For this review, use the dimensioned drawing (mm, ordinates from the lowest corner) and the shaded views. A direction names the side the tool comes from. Coordinates: 2 decimals unless noted, no trailing zeros. Loops run counter-clockwise (first coordinate to the right, second up) from the corner with the lowest first, then second, coordinate; pieces in that order, holes last. Notation, with made-up numbers: (7.25, 64.5) - (24.25, 64.5) arc R16 cw to (24.25, 91.5) - close; hole circle Ø8 at (54.5, -5.75). An arc over 180 degrees is marked (long way). Answer in a Markdown table with one row per item. Add a question column.
(1) Machinability: for the marked faces 5, 6, 7 and 8, which of the approach directions +Z, -Z, +X, -X, +Y, -Y give a long, thin tool a straight path to every point of the face, cutting with its end or side? Answer none if there is none.
(2) For line 1 along Y through (x, z) = (2, 7.75); line 2 along X through (y, z) = (47.5, 9), list the stretches that pass through material, from the lowest coordinate up.
(3) We need section B-B on z = 3. Write out the cut boundary in (x, y), plus the area to 3 significant figures.
(4) Mouldability with a two-part tool opening along Y and no side actions: class the marked faces 1, 2, 3 and 4 as +Y half, -Y half, draft (parallel to the pull), parting line (faces both ways), or undercut.
(5) We need section A-A on x = 3. Write out the cut boundary in (y, z), plus the area to 3 significant figures.
(6) We need section C-C on z = 7.25. Write out the cut boundary in (x, y).
(7) We need section D-D on y = 43. Write out the cut boundary in (x, z), plus the area to 3 significant figures.
(8) For P1, Ø1.5, axis at x = 16.5, z = 11, coming from the +Y side; P2, Ø5.5, axis at y = 48.5, z = 11.5, coming from the +X side; P3, Ø5.5, axis at x = 1.5, y = 40, coming from the -Z side, all flat-tipped, find the tip position at first contact; note any pin that passes through.
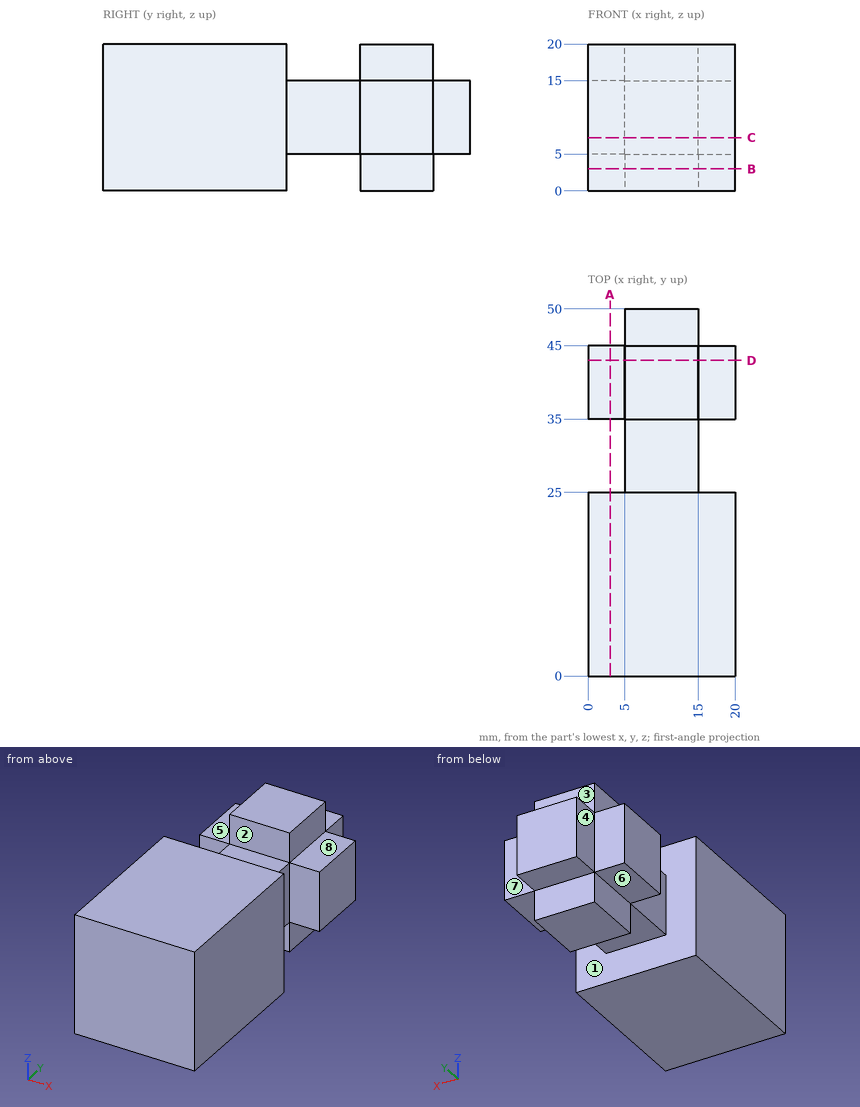
Outcome:
| question | item | result |
|---|---|---|
| 1 | face 5 | +Z, -X, +Y |
| 1 | face 6 | -Z, -X, +Y |
| 1 | face 7 | +Z, -Z, +X, +Y |
| 1 | face 8 | +Z, +X, +Y |
| 2 | line 1 | 0 to 25, 35 to 45 |
| 2 | line 2 | 5 to 15 |
| 3 | outline | (0, 0) - (20, 0) - (20, 25) - (0, 25) - close; (5, 35) - (15, 35) - (15, 45) - (5, 45) - close |
| 3 | area | 600 mm² |
| 4 | face 1 | undercut |
| 4 | face 2 | undercut |
| 4 | face 3 | +Y half |
| 4 | face 4 | draft |
| 5 | outline | (0, 0) - (25, 0) - (25, 20) - (0, 20) - close; (35, 5) - (45, 5) - (45, 15) - (35, 15) - close |
| 5 | area | 600 mm² |
| 6 | outline | (0, 0) - (20, 0) - (20, 25) - (15, 25) - (15, 35) - (20, 35) - (20, 45) - (15, 45) - (15, 50) - (5, 50) - (5, 45) - (0, 45) - (0, 35) - (5, 35) - (5, 25) - (0, 25) - close |
| 7 | outline | (0, 5) - (5, 5) - (5, 0) - (15, 0) - (15, 5) - (20, 5) - (20, 15) - (15, 15) - (15, 20) - (5, 20) - (5, 15) - (0, 15) - close |
| 7 | area | 300 mm² |
| 8 | P1 | y = 45 |
| 8 | P2 | x = 15 |
| 8 | P3 | z = 5 |
